Read the model definition and answer for the solid it produces. Units are mm, in the model's axes. Face numbers are marked on the shaded views. Coordinates: 2 decimals unless noted, no trailing zeros. Loops run counter-clockwise (first coordinate to the right, second up) from the corner with the lowest first, then second, coordinate; pieces in that order, holes last. Notation, with made-up numbers: (87.5, -20.5) -> (143.5, -20.5) arc R19 ccw to (143.5, -16.5) -> close; hole circle Ø4 at (80, -33.5). An arc over 180 degrees is marked (long way). Answer in a Markdown table with one row per item.
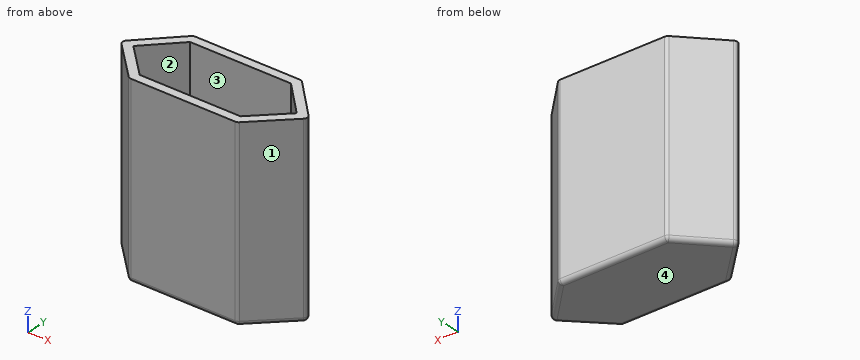
```python
from build123d import *

# Parameters (mm, degrees)
F1_DEPTH     = 42
F2_DEPTH     = 2
F3_R         = 1
F4_T1_DEPTH  = 43.446869231
F4_T3_DEPTH  = 42.0361861213
F4_T5_DEPTH  = 42.0250945478
F4_T7_DEPTH  = 43.4842607953
F4_T9_DEPTH  = 42.0552929075
F4_T11_DEPTH = 42.0664740253
F4_T16_DEPTH = 1
F4_T22_DEPTH = 1
F4_T28_DEPTH = 1
F4_T34_DEPTH = 1
F4_T40_DEPTH = 1
F4_T46_DEPTH = 1


# Not quite as in the source:
# - a fillet or chamfer that OpenCascade refuses, or shapes differently, is made with other operations: its cross-section is extruded or revolved along the edge and cut away or added


with BuildPart() as f1:
    # F0 (on Top) → F1 (new body)
    with BuildSketch(Plane.XY):
        Polygon((-6.2833941388, -9.0027643815), (2.8193882778, -0.0290314764), (-6.2592354511, 9.2972356185), (-30.6566489974, 9.2972356185), (-39.5983849299, -0.0288091293), (-30.6324186742, -9.0027643815), align=None)
        Polygon((-7.1034697771, 7.2972356185), (0, 0), (-7.1034697771, -7.0027643815), (-29.8034697771, -7.0027643815), (-36.8, 0), (-29.8034697771, 7.2972356185), align=None, mode=Mode.SUBTRACT)
    extrude(amount=F1_DEPTH)

    # F0 (on Top) → F2 (join)
    with BuildSketch(Plane.XY):
        Polygon((-7.1034697771, -7.0027643815), (0, 0), (-7.1034697771, 7.2972356185), (-29.8034697771, 7.2972356185), (-36.8, 0), (-29.8034697771, -7.0027643815), align=None)
    extrude(amount=F2_DEPTH)

    # F3
    f3_edges = [f1.edges().sort_by_distance(p)[0] for p in [
        (-1.719924, 4.634102, 0),
        (-18.457942, 9.297236, 0),
        (-35.127517, 4.634213, 0),
        (-35.115402, -4.515787, 0),
        (-18.457906, -9.002764, 0),
        (-1.732003, -4.515898, 0),
    ]]
    fillet(f3_edges, radius=F3_R)

    # F4: fillet of radius 1 on 6 edges, made by hand

    # F4_s2 → F4_t1 (cut)
    with BuildSketch(Plane.XY.offset(1)):
        with BuildLine():
            ThreePointArc((-38.9066140644, -0.7211963873), (-39.1991394765, -0.0246989321), (-38.9210153062, 0.6776733109))
            Line((-38.9210153062, 0.6776733109), (-39.5983849299, -0.0288091293))
            Line((-39.5983849299, -0.0288091293), (-38.9066140644, -0.7211963873))
        make_face()
    extrude(amount=F4_T1_DEPTH, mode=Mode.SUBTRACT)

    # F4_s4 → F4_t3 (cut)
    with BuildSketch(Plane.XY.offset(1)):
        with BuildLine():
            ThreePointArc((-30.2179442256, -9.0027643815), (-30.6008333593, -8.9265586829), (-30.9253658251, -8.7095562041))
            Line((-30.9253658251, -8.7095562041), (-30.6324186742, -9.0027643815))
            Line((-30.6324186742, -9.0027643815), (-30.2179442256, -9.0027643815))
        make_face()
    extrude(amount=F4_T3_DEPTH, mode=Mode.SUBTRACT)

    # F4_s6 → F4_t5 (cut)
    with BuildSketch(Plane.XY.offset(1)):
        with BuildLine():
            ThreePointArc((-5.9913911517, -8.7149011003), (-6.3140487209, -8.9280040042), (-6.693431958, -9.0027643815))
            Line((-6.693431958, -9.0027643815), (-6.2833941388, -9.0027643815))
            Line((-6.2833941388, -9.0027643815), (-5.9913911517, -8.7149011003))
        make_face()
    extrude(amount=F4_T5_DEPTH, mode=Mode.SUBTRACT)

    # F4_s8 → F4_t7 (cut)
    with BuildSketch(Plane.XY.offset(1)):
        with BuildLine():
            ThreePointArc((2.1117349451, -0.726652457), (2.4096411281, -0.0248122758), (2.1262503938, 0.6830135684))
            Line((2.1262503938, 0.6830135684), (2.8193882778, -0.0290314764))
            Line((2.8193882778, -0.0290314764), (2.1117349451, -0.726652457))
        make_face()
    extrude(amount=F4_T7_DEPTH, mode=Mode.SUBTRACT)

    # F4_s10 → F4_t9 (cut)
    with BuildSketch(Plane.XY.offset(1)):
        with BuildLine():
            ThreePointArc((-5.9647963592, 8.9947649251), (-6.2924627239, 9.2185198598), (-6.6813526141, 9.2972356185))
            Line((-6.6813526141, 9.2972356185), (-6.2592354511, 9.2972356185))
            Line((-6.2592354511, 9.2972356185), (-5.9647963592, 8.9947649251))
        make_face()
    extrude(amount=F4_T9_DEPTH, mode=Mode.SUBTRACT)

    # F4_s12 → F4_t11 (cut)
    with BuildSketch(Plane.XY.offset(1)):
        with BuildLine():
            ThreePointArc((-30.2300593872, 9.2972356185), (-30.6224381102, 9.2170393681), (-30.9518822285, 8.9893134941))
            Line((-30.9518822285, 8.9893134941), (-30.6566489974, 9.2972356185))
            Line((-30.6566489974, 9.2972356185), (-30.2300593872, 9.2972356185))
        make_face()
    extrude(amount=F4_T11_DEPTH, mode=Mode.SUBTRACT)


with BuildPart() as f4_tool14:
    # F4_s15 → F4_t16 (new body)
    with BuildSketch(Plane.XY.offset(1)):
        Polygon((-30.2300593872, 8.2972356185), (-30.2300593872, 9.2972356185), (-30.6566489974, 9.2972356185), (-30.9518822285, 8.9893134941), align=None)
    extrude(amount=-F4_T16_DEPTH)

    # F4_s17 → F4_t18 (revolve, cut)
    with BuildSketch(Plane(origin=(-30.2300593872, 8.2972356185, 1), x_dir=(0.3923787229, -0.9198037496, 0), z_dir=(0.9198037496, 0.3923787229, 0))):
        with BuildLine():
            ThreePointArc((0, -1), (1, 0), (0, 1))
            Line((0, 1), (0, -1))
        make_face()
    revolve(axis=Axis((-30.2300593872, 8.2972356185, 1), (0, 0, -1)), mode=Mode.SUBTRACT)


with BuildPart() as f1_1:
    add(f1.part)

    # F4_t13: cut F4_tool14
    add(f4_tool14.part, mode=Mode.SUBTRACT)


with BuildPart() as f4_tool20:
    # F4_s21 → F4_t22 (new body)
    with BuildSketch(Plane.XY.offset(1)):
        Polygon((-6.6813526141, 8.2972356185), (-5.9647963592, 8.9947649251), (-6.2592354511, 9.2972356185), (-6.6813526141, 9.2972356185), align=None)
    extrude(amount=-F4_T22_DEPTH)

    # F4_s23 → F4_t24 (revolve, cut)
    with BuildSketch(Plane(origin=(-6.6813526141, 8.2972356185, 1), x_dir=(-0.3888898902, -0.9212842413, 0), z_dir=(0.9212842413, -0.3888898902, 0))):
        with BuildLine():
            ThreePointArc((0, -1), (1, 0), (0, 1))
            Line((0, 1), (0, -1))
        make_face()
    revolve(axis=Axis((-6.6813526141, 8.2972356185, 1), (0, 0, -1)), mode=Mode.SUBTRACT)


with BuildPart() as f1_2:
    add(f1_1.part)

    # F4_t19: cut F4_tool20
    add(f4_tool20.part, mode=Mode.SUBTRACT)


with BuildPart() as f4_tool26:
    # F4_s27 → F4_t28 (new body)
    with BuildSketch(Plane.XY.offset(1)):
        Polygon((1.4096941389, -0.0145157382), (2.1117349451, -0.726652457), (2.8193882778, -0.0290314764), (2.1262503938, 0.6830135684), align=None)
    extrude(amount=-F4_T28_DEPTH)

    # F4_s29 → F4_t30 (revolve, cut)
    with BuildSketch(Plane(origin=(1.4096941389, -0.0145157382, 1), x_dir=(-0.9999469893, 0.0102965376, 0), z_dir=(-0.0102965376, -0.9999469893, 0))):
        with BuildLine():
            ThreePointArc((0, -1), (1, 0), (0, 1))
            Line((0, 1), (0, -1))
        make_face()
    revolve(axis=Axis((1.4096941389, -0.0145157382, 1), (0, 0, -1)), mode=Mode.SUBTRACT)


with BuildPart() as f1_3:
    add(f1_2.part)

    # F4_t25: cut F4_tool26
    add(f4_tool26.part, mode=Mode.SUBTRACT)


with BuildPart() as f4_tool32:
    # F4_s33 → F4_t34 (new body)
    with BuildSketch(Plane.XY.offset(1)):
        Polygon((-6.693431958, -8.0027643815), (-5.9913911517, -8.7149011003), (-6.2833941388, -9.0027643815), (-6.693431958, -9.0027643815), align=None)
    extrude(amount=-F4_T34_DEPTH)

    # F4_s35 → F4_t36 (revolve, cut)
    with BuildSketch(Plane(origin=(-6.693431958, -8.0027643815, 1), x_dir=(-0.3793832371, 0.9252396227, 0), z_dir=(-0.9252396227, -0.3793832371, 0))):
        with BuildLine():
            ThreePointArc((0, -1), (1, 0), (0, 1))
            Line((0, 1), (0, -1))
        make_face()
    revolve(axis=Axis((-6.693431958, -8.0027643815, 1), (0, 0, -1)), mode=Mode.SUBTRACT)


with BuildPart() as f1_4:
    add(f1_3.part)

    # F4_t31: cut F4_tool32
    add(f4_tool32.part, mode=Mode.SUBTRACT)


with BuildPart() as f4_tool38:
    # F4_s39 → F4_t40 (new body)
    with BuildSketch(Plane.XY.offset(1)):
        Polygon((-30.2179442256, -8.0027643815), (-30.2179442256, -9.0027643815), (-30.6324186742, -9.0027643815), (-30.9253658251, -8.7095562041), align=None)
    extrude(amount=-F4_T40_DEPTH)

    # F4_s41 → F4_t42 (revolve, cut)
    with BuildSketch(Plane(origin=(-30.2179442256, -8.0027643815, 1), x_dir=(0.3828891336, 0.9237943014, 0), z_dir=(-0.9237943014, 0.3828891336, 0))):
        with BuildLine():
            ThreePointArc((0, -1), (1, 0), (0, 1))
            Line((0, 1), (0, -1))
        make_face()
    revolve(axis=Axis((-30.2179442256, -8.0027643815, 1), (0, 0, -1)), mode=Mode.SUBTRACT)


with BuildPart() as f1_5:
    add(f1_4.part)

    # F4_t37: cut F4_tool38
    add(f4_tool38.part, mode=Mode.SUBTRACT)


with BuildPart() as f4_tool44:
    # F4_s45 → F4_t46 (new body)
    with BuildSketch(Plane.XY.offset(1)):
        Polygon((-38.1991924649, -0.0144045646), (-38.9066140644, -0.7211963873), (-39.5983849299, -0.0288091293), (-38.9210153062, 0.6776733109), align=None)
    extrude(amount=-F4_T46_DEPTH)

    # F4_s47 → F4_t48 (revolve, cut)
    with BuildSketch(Plane(origin=(-38.1991924649, -0.0144045646, 1), x_dir=(0.9999470116, 0.0102943674, 0), z_dir=(-0.0102943674, 0.9999470116, 0))):
        with BuildLine():
            ThreePointArc((0, -1), (1, 0), (0, 1))
            Line((0, 1), (0, -1))
        make_face()
    revolve(axis=Axis((-38.1991924649, -0.0144045646, 1), (0, 0, -1)), mode=Mode.SUBTRACT)


with BuildPart() as f1_6:
    add(f1_5.part)

    # F4_t43: cut F4_tool44
    add(f4_tool44.part, mode=Mode.SUBTRACT)


solid = f1_6.part
```
1. Given pin 1 Ø3 at (x, z) = (-33, 16.5) entering from -Y; pin 2 Ø6 at (x, y) = (-7, 2.5) entering from +Z; pin 3 Ø1 at (y, z) = (3, 24) entering from +X, each flat-ended and moving along its own axis, determine where each tip first touches the part or whether it passes through.
A:
| item | result |
|---|---|
| pin 1 | stops at y = -8.13 |
| pin 2 | stops at z = 2 |
| pin 3 | stops at x = 0.36 |
2. The mould has two halves that part along X. Classify the marked faces 1, 2, 3 and 4: pulls with the +X half, pulls with the -X half, needs draft (parallel to the pull), parting line crosses it, or undercut.
A:
| item | result |
|---|---|
| face 1 | pulls with the +X half |
| face 2 | undercut |
| face 3 | undercut |
| face 4 | needs draft |
3. Find the intervals of material crossed by probe 1 along Y at (x, z) = (-17, 25); probe 2 along Z at (x, y) = (-18, -4); probe 3 along Y at (x, z) = (-35, 3), in increasing order.
A:
| item | result |
|---|---|
| probe 1 | y = -9 to -7, 7.3 to 9.3 |
| probe 2 | z = 0 to 2 |
| probe 3 | y = -4.63 to -1.8, 1.88 to 4.77 |
4. A cutting plane is placed at B-B on z = 29. Give the vertices of the cut face in (x, y).
A:
| item | result |
|---|---|
| outline | (-38.92, 0.68) arc R1 ccw to (-38.91, -0.72) -> (-30.93, -8.71) arc R1 ccw to (-30.22, -9) -> (-6.69, -9) arc R1 ccw to (-5.99, -8.71) -> (2.11, -0.73) arc R1 ccw to (2.13, 0.68) -> (-5.96, 8.99) arc R1 ccw to (-6.68, 9.3) -> (-30.23, 9.3) arc R1 ccw to (-30.95, 8.99) -> close; hole (-36.8, 0) -> (-29.8, -7) -> (-7.1, -7) -> (0, 0) -> (-7.1, 7.3) -> (-29.8, 7.3) -> close |
5. A cutting plane is placed at A-A on x = -20.5. Give the vertices of the cut face in (y, z).
A:
| item | result |
|---|---|
| outline | (-9, 1) arc R1 ccw to (-8, 0) -> (8.3, 0) arc R1 ccw to (9.3, 1) -> (9.3, 42) -> (7.3, 42) -> (7.3, 2) -> (-7, 2) -> (-7, 42) -> (-9, 42) -> close |
